Part print with two shaded views. Sizes in mm from the minimum x, y, z corner. A direction names the side the tool comes from. Coordinates: 2 decimals unless noted, no trailing zeros. Write each loop counter-clockwise with the first axis right and the second up, starting at its lowest first coordinate (ties: lowest second). Pieces come first, ordered by that corner, then holes.
Q1. Band-saw the part on B-B, the plane x = 122.5. Write the cut outline in (y, z), plus the area to 3 significant figures.
Q2. Pin check, flat tips, straight feed: P1, Ø1.5, axis at y = 64.5, z = 16, coming from the +X side; P2, Ø3, axis at x = 75.5, z = 15.5, coming from the -Y side; P3, Ø4.5, axis at x = 122.5, y = 20, coming from the +Z side; P4, Ø10, axis at y = 51, z = 24, coming from the -X side. Stop position of each tip, or through.
Q3. Which spindle directions (+Z, -Z, +X, -X, +Y, -Y) get a long thin tool onto all of the face, cutting with end or side? Do the marked faces 1, 2 and 3. Say none if no direction does.
Q4. Band-saw the part on A-A, the plane y = 20. Write the cut outline in (x, z).
Q5. Band-saw the part on C-C, the plane z = 7.75. Write the cut outline in (x, y), plus the area to 3 significant figures.
Q6. Band-saw the part on D-D, the plane x = 181. Write the cut outline in (y, z).
Q7. Drill centre lines: probe 1 along Z at (x, y) = (60, 137.5); probe 2 along Z at (x, y) = (150, 137); probe 3 along Y at (x, z) = (198, 2.75). Where is each one in solid material? Low to high.
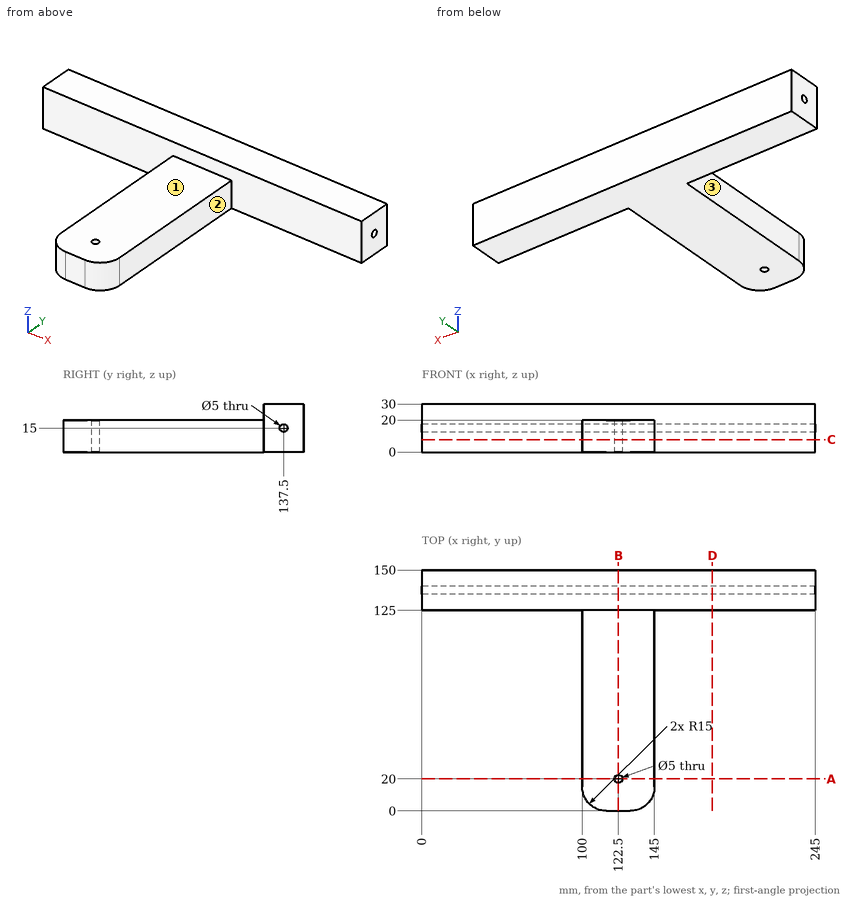
Answer sheet:
1. outline: (0, 0) - (17.5, 0) - (17.5, 20) - (0, 20) - close; (22.5, 0) - (150, 0) - (150, 30) - (125, 30) - (125, 20) - (22.5, 20) - close; hole circle Ø5 at (137.5, 15)
1. area: 3,130 mm2
2. P1: stops at x = 145
2. P2: stops at y = 125
2. P3: passes through
2. P4: stops at x = 100
3. face 1: +Z, +X, -X, -Y
3. face 2: +Z, -Z, +X, -Y
3. face 3: +Z, -Z, -X, -Y
4. outline: (100, 0) - (120, 0) - (120, 20) - (100, 20) - close; (125, 0) - (145, 0) - (145, 20) - (125, 20) - close
5. outline: (0, 125) - (100, 125) - (100, 15) arc R15 ccw to (115, 0) - (130, 0) arc R15 ccw to (145, 15) - (145, 125) - (245, 125) - (245, 150) - (0, 150) - close; hole circle Ø5 at (122.5, 20)
5. area: 11,600 mm2
6. outline: (125, 0) - (150, 0) - (150, 30) - (125, 30) - close; hole circle Ø5 at (137.5, 15)
7. probe 1: z = 0 to 12.5, 17.5 to 30
7. probe 2: z = 0 to 12.55, 17.45 to 30
7. probe 3: y = 125 to 150
